Could you check a few things on this drawing? It's one solid part, dimensions in mm from its lowest x, y, z. Coordinates: 2 decimals unless noted, no trailing zeros. Write each loop counter-clockwise with the first axis right and the second up, starting at its lowest first coordinate (ties: lowest second). Pieces come first, ordered by that corner, then holes. Notation, with made-up numbers: M 67.5,86 L 113.5,86 A13 cw 113.5,97 Z; hole C 5,67.5 d2. An arc over 180 degrees is marked long. Use a Markdown table: item, result.
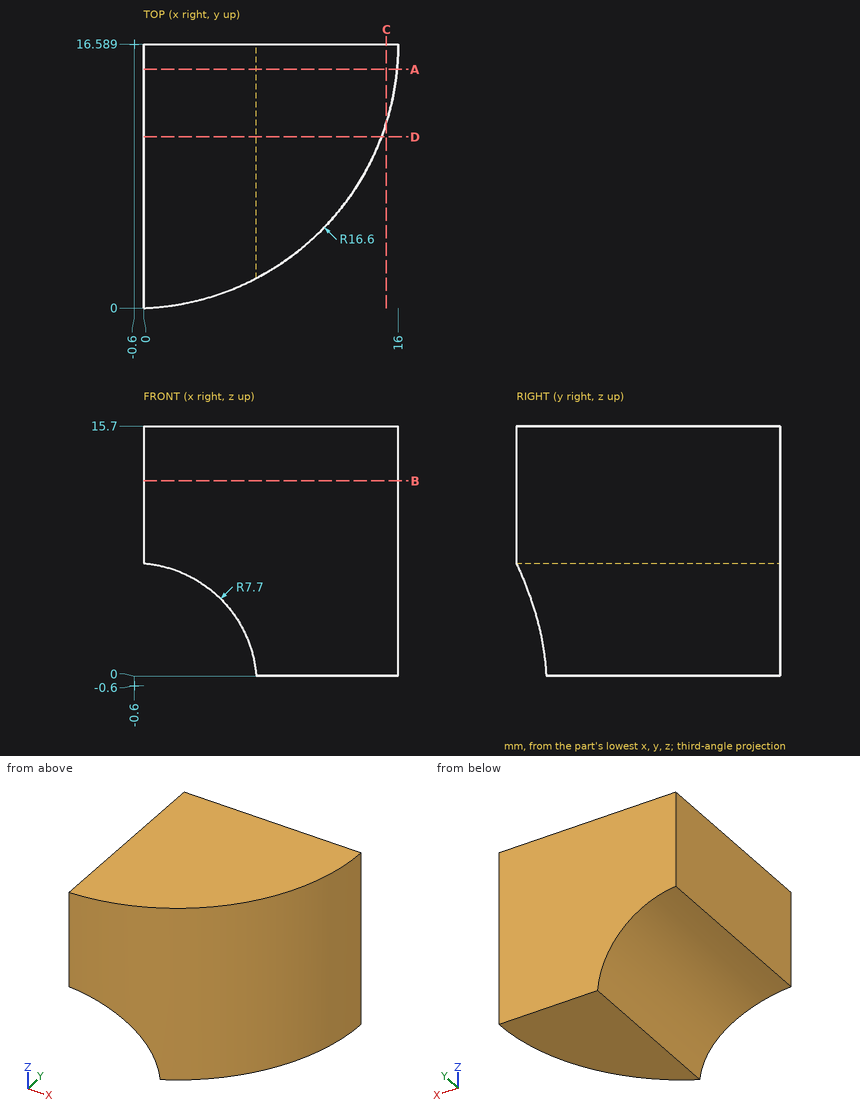
1. Suppose I cut it at B-B on z = 12.25. Write out the boundary of the cut face in (x, y), and give its area (3 significant figures).
Answers follow:
| item | result |
|---|---|
| outline | M 0,0 A16.6 ccw 16,16.59 L 0,16.59 Z |
| area | 206 mm2 |
2. Will these pins go through, and if not, where does the flat tip stop? pin 1 Ø1.5 at (y, z) = (2, 13) entering from +X; pin 2 Ø5 at (y, z) = (13, 7) entering from +X; pin 3 Ø5 at (y, z) = (11, 3) entering from +X.
Answers follow:
| item | result |
|---|---|
| pin 1 | stops at x = 8.57 |
| pin 2 | stops at x = 15.96 |
| pin 3 | stops at x = 15.71 |
3. I need wall thicknesses on probe 1 along Y at (x, z) = (13, 2); probe 2 along Y at (x, z) = (5.25, 15.25); probe 3 along X at (y, z) = (3, 8.25) (1 decimal). Which ranges of each line are inside material? Lowest first, please.
Answers follow:
| item | result |
|---|---|
| probe 1 | y = 7.07 to 16.59 |
| probe 2 | y = 1.05 to 16.59 |
| probe 3 | x = 0 to 8.9 |
4. Suppose I cut it at C-C on x = 15.25. Write out the boundary of the cut face in (y, z).
Answers follow:
| item | result |
|---|---|
| outline | M 11.66,0 L 16.59,0 L 16.59,15.7 L 11.66,15.7 Z |
5. Suppose I cut it at D-D on y = 10.75. Write out the boundary of the cut face in (x, z).
Answers follow:
| item | result |
|---|---|
| outline | M 0,7.08 A7.7 cw 7.08,0 L 14.94,0 L 14.94,15.7 L 0,15.7 Z |
6. Suppose I cut it at A-A on y = 15. Write out the boundary of the cut face in (x, z).
Answers follow:
| item | result |
|---|---|
| outline | M 0,7.08 A7.7 cw 7.08,0 L 15.92,0 L 15.92,15.7 L 0,15.7 Z |
